Could you check a few things on this model? Use its own coordinates, in mm. Face numbers are marked on the shaded views. A direction names the side the tool comes from. Round coordinates to 2 decimals unless told otherwise and drop trailing zeros. Write each loop counter-clockwise with the first axis right and the second up, starting at its lowest first coordinate (ties: lowest second). Pieces come first, ordered by that corner, then holes. Notation, with made-up numbers: M 42.5,88.5 L 98.5,88.5 A20 ccw 98.5,123.5 Z; hole C 2,68 d6. An arc over 180 degrees is marked long. One line per item, written item: value. Start each with the question number.
(1) I want a section at B-B on x = 20. Please give me the cut outline in (y, z).
(2) If I drill on L1, parallel to Z at x = 28, y = -212; L2, parallel to X at y = -224.5, z = 13.5; L3, parallel to Z at x = 3.5, y = -66, over which ranges is the centre line in solid material (lowest first)?
(3) I want a section at A-A on y = -98.5. Please give me the cut outline in (x, z).
(4) Which directions (+Z, -Z, +X, -X, +Y, -Y) give clear straight access to the entire face, cutting with the end or side of a thin tool? Please do the marked faces 1 and 2.
(5) I'm going to push a flat-ended pin straight in: pin 1 Ø14.5 at (x, y) = (27, -212.5) entering from +Z. Where does the tip first touch, or does it pass through?
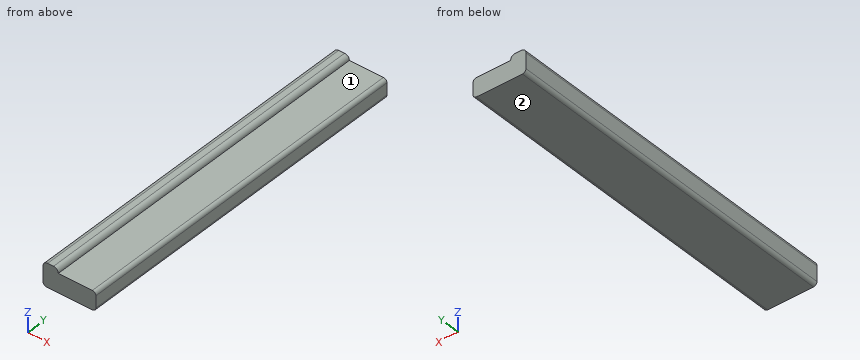
```python
from build123d import *

# Parameters (mm, degrees)
F1_DEPTH = 300


with BuildPart() as f1:
    # F0 (on Front) → F1 (new body)
    with BuildSketch(Plane.XZ):
        with BuildLine():
            ThreePointArc((0, 3), (0.87868, 0.87868), (3, 0))
            Line((3, 0), (42, 0))
            ThreePointArc((42, 0), (44.12132, 0.87868), (45, 3))
            Line((45, 3), (45, 13))
            ThreePointArc((45, 13), (44.12132, 15.12132), (42, 16))
            Line((42, 16), (13, 16))
            ThreePointArc((13, 16), (11.828427, 18.828427), (9, 20))
            Line((9, 20), (4, 20))
            ThreePointArc((4, 20), (1.171573, 18.828427), (0, 16))
            Line((0, 16), (0, 3))
        make_face()
    extrude(amount=F1_DEPTH)


solid = f1.part
```
Found:
1. outline: M -300,0 L 0,0 L 0,16 L -300,16 Z
2. L1: z = 0 to 16
2. L2: x = 0 to 44.96
2. L3: z = 0 to 19.97
3. outline: M 0,3 A3 ccw 3,0 L 42,0 A3 ccw 45,3 L 45,13 A3 ccw 42,16 L 13,16 A4 ccw 9,20 L 4,20 A4 ccw 0,16 Z
4. face 1: +Z, +X, +Y, -Y
4. face 2: -Z, +X, -X, +Y, -Y
5. pin 1: stops at z = 16
